Could you check a few things on this drawing? It's one solid part, dimensions in mm from its lowest x, y, z. Coordinates: 2 decimals unless noted, no trailing zeros. Order: outer loops, then holes, each group sorted by start corner. A loop starts at its lowest first (then second) coordinate and runs counter-clockwise, first axis right, second up. Notation, with made-up numbers: (78, -40) - (126, -40) arc R33 ccw to (126, -5) - close; hole circle Ø3 at (9.5, 64.5). An arc over 180 degrees is marked (long way). Answer in a Markdown table with one row per item. Add a question column.
Item 1: I want a section at B-B (z = 165.1). Please give me the cut outline in (x, y).
Item 2: Will these pins go through, and if not, where does the flat tip stop? pin 1 Ø1.5 at (y, z) = (1, 286) entering from +X; pin 2 Ø2 at (x, y) = (133, 3) entering from -Z.
Item 3: I want a section at A-A (x = 165.1). Please give me the cut outline in (y, z), plus the area to 3 significant figures.
Item 4: I want a section at C-C (y = 3.75). Please give me the cut outline in (x, z), plus the area to 3 significant figures.
Item 5: If I drill on line 1 along X through (y, z) = (1, 168.5); line 2 along X through (y, z) = (5.25, 165.1), over which ranges is the centre line in solid material (lowest first)? Write a range as from..to.
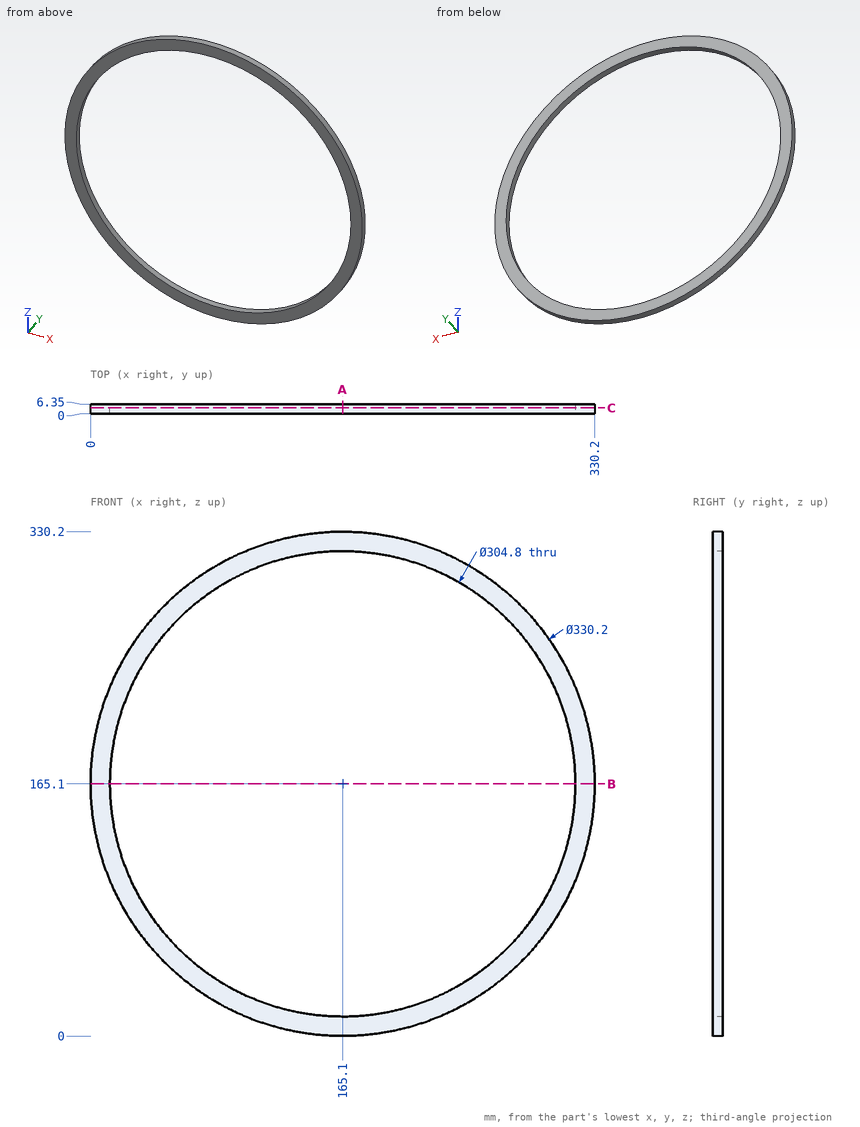
Values follow:
| question | item | result |
|---|---|---|
| 1 | outline | (0, 0) - (12.7, 0) - (12.7, 6.35) - (0, 6.35) - close; (317.5, 0) - (330.2, 0) - (330.2, 6.35) - (317.5, 6.35) - close |
| 2 | pin 1 | stops at x = 278.33 |
| 2 | pin 2 | stops at z = 2.96 |
| 3 | outline | (0, 0) - (6.35, 0) - (6.35, 12.7) - (0, 12.7) - close; (0, 317.5) - (6.35, 317.5) - (6.35, 330.2) - (0, 330.2) - close |
| 3 | area | 161 mm^2 |
| 4 | outline | circle Ø330.2 at (165.1, 165.1); hole circle Ø304.8 at (165.1, 165.1) |
| 4 | area | 12,700 mm^2 |
| 5 | line 1 | x = 0.04..12.74, 317.46..330.16 |
| 5 | line 2 | x = 0..12.7, 317.5..330.2 |
